Here's how the part is built. I have some questions about the finished solid (model axes, mm). A direction names the side the tool comes from. Round coordinates to 2 decimals unless told otherwise and drop trailing zeros. Loops run counter-clockwise (first coordinate to the right, second up) from the corner with the lowest first, then second, coordinate; pieces in that order, holes last. Notation, with made-up numbers: M -16,1 L 40,1 A16 ccw 40,17 Z; hole C 34.5,1 d9. An arc over 180 degrees is marked long. Answer as a JSON object with one key per item and string values.
from build123d import *

# Parameters (mm, degrees)
SKETCH1_R           = 2.1
SKETCH1_R_2         = 10
BOSS_EXTRUDE1_DEPTH = 6.35


with BuildPart() as part:
    # Sketch1 → Boss-Extrude1 (new body)
    with BuildSketch(Plane(origin=(0, 0, 0), x_dir=(1, 0, 0), z_dir=(0, 1, 0))):
        with BuildLine():
            ThreePointArc((-138, 42.5), (-180.5, 0), (-138, -42.5))
            Line((-138, -42.5), (0, -42.5))
            ThreePointArc((0, -42.5), (42.5, 0), (0, 42.5))
            Line((0, 42.5), (-138, 42.5))
        make_face()
        with BuildLine():
            Line((-103, 2.5), (-93, 2.5))
            ThreePointArc((-93, 2.5), (-90.5, 0), (-93, -2.5))
            Line((-93, -2.5), (-103, -2.5))
            ThreePointArc((-103, -2.5), (-105.5, 0), (-103, 2.5))
        make_face(mode=Mode.SUBTRACT)
        with BuildLine():
            ThreePointArc((-138, -37.5), (-140.5, -35), (-138, -32.5))
            Line((-138, -32.5), (-128, -32.5))
            ThreePointArc((-128, -32.5), (-125.5, -35), (-128, -37.5))
            Line((-128, -37.5), (-138, -37.5))
        make_face(mode=Mode.SUBTRACT)
        with BuildLine():
            ThreePointArc((-173, -2.5), (-175.5, 0), (-173, 2.5))
            Line((-173, 2.5), (-163, 2.5))
            ThreePointArc((-163, 2.5), (-160.5, 0), (-163, -2.5))
            Line((-163, -2.5), (-173, -2.5))
        make_face(mode=Mode.SUBTRACT)
        with BuildLine():
            ThreePointArc((-138, -10), (-148, 0), (-138, 10))
            Line((-138, 10), (-128, 10))
            ThreePointArc((-128, 10), (-118, 0), (-128, -10))
            Line((-128, -10), (-138, -10))
        make_face(mode=Mode.SUBTRACT)
        with BuildLine():
            ThreePointArc((-138, 32.5), (-140.5, 35), (-138, 37.5))
            Line((-138, 37.5), (-128, 37.5))
            ThreePointArc((-128, 37.5), (-125.5, 35), (-128, 32.5))
            Line((-128, 32.5), (-138, 32.5))
        make_face(mode=Mode.SUBTRACT)
        with Locations(Location((0, 35, 0), (0, 0, 270))):
            Circle(SKETCH1_R, mode=Mode.SUBTRACT)
        with Locations(Location((0, -35, 0), (0, 0, 270))):
            Circle(SKETCH1_R, mode=Mode.SUBTRACT)
        with Locations(Location((-17.67766953, -17.67766953, 0), (0, 0, 270))):
            Circle(SKETCH1_R, mode=Mode.SUBTRACT)
        with Locations(Location((17.67766953, -17.67766953, 0), (0, 0, 270))):
            Circle(SKETCH1_R, mode=Mode.SUBTRACT)
        with Locations(Location((-35, 0, 0), (0, 0, 270))):
            Circle(SKETCH1_R, mode=Mode.SUBTRACT)
        with Locations(Location((-17.67766953, 17.67766953, 0), (0, 0, 270))):
            Circle(SKETCH1_R, mode=Mode.SUBTRACT)
        with Locations(Location((0, 0, 0), (0, 0, 270))):
            Circle(SKETCH1_R_2, mode=Mode.SUBTRACT)
        with Locations(Location((35, 0, 0), (0, 0, 270))):
            Circle(SKETCH1_R, mode=Mode.SUBTRACT)
        with Locations(Location((17.67766953, 17.67766953, 0), (0, 0, 270))):
            Circle(SKETCH1_R, mode=Mode.SUBTRACT)
    extrude(amount=-BOSS_EXTRUDE1_DEPTH)


solid = part.part
Item 1: For faces 4 (the face through (-140.5, -3.1, 35.1)), 5 (the face through (-71, -6.35, -1)), which set-ups out of +Z, -Z, +X, -X, +Y, -Y let a thin tool reach every point of the face, with its end or its side?
Solution:
{"face 4": "+Y, -Y", "face 5": "+Z, -Z, +X, -X, -Y"}
Item 2: I want a section at A-A on z = 0. List the corners of the cut face in (x, y) for me, plus the area to 3 significant figures.
Solution:
{"outline": "M -180.5,-6.35 L -175.5,-6.35 L -175.5,0 L -180.5,0 Z; M -160.5,-6.35 L -148,-6.35 L -148,0 L -160.5,0 Z; M -118,-6.35 L -105.5,-6.35 L -105.5,0 L -118,0 Z; M -90.5,-6.35 L -37.1,-6.35 L -37.1,0 L -90.5,0 Z; M -32.9,-6.35 L -10,-6.35 L -10,0 L -32.9,0 Z; M 10,-6.35 L 32.9,-6.35 L 32.9,0 L 10,0 Z; M 37.1,-6.35 L 42.5,-6.35 L 42.5,0 L 37.1,0 Z", "area": "855 mm2"}
Item 3: If I drill on L1, parallel to X at y = -3.5, z = 7.5; L2, parallel to X at y = -1.5, z = 3; L3, parallel to Z at x = -147, y = -2.25, over which ranges is the centre line in solid material (lowest first)? Write a range as from..to.
Solution:
{"L1": "x = -179.83..-144.61, -121.39..-6.61, 6.61..41.83", "L2": "x = -180.39..-147.54, -118.46..-9.54, 9.54..42.39", "L3": "z = -41.54..-4.36, 4.36..41.54"}
Item 4: We'd pull the mould along Z, two halves only. Please class faces 1 (the face through (-71, 0, -1)), 2 (the face through (0.09, -3.13, 32.9)), 3 (the face through (-180.49, -3.13, -0.93)): +Z half, -Z half, draft (parallel to the pull), parting line (faces both ways), or undercut.
Solution:
{"face 1": "draft", "face 2": "undercut", "face 3": "parting line"}
Item 5: For P1, Ø1, axis at y = -4, z = -16.5, coming from the +X side; P2, Ø1.9, axis at x = -167.5, y = -3.5, coming from the -Z side, each with a flat end and sliding along its axis, tell me the tip position at first contact or that it passes through.
Solution:
{"P1": "stops at x = 39.37", "P2": "stops at z = -31.48"}
Item 6: I want a section at D-D on z = 35. List the corners of the cut face in (x, y) for me.
Solution:
{"outline": "M -162.11,-6.35 L -140.5,-6.35 L -140.5,0 L -162.11,0 Z; M -125.5,-6.35 L -2.1,-6.35 L -2.1,0 L -125.5,0 Z; M 2.1,-6.35 L 24.11,-6.35 L 24.11,0 L 2.1,0 Z"}
Item 7: I want a section at B-B on x = -97.5. List the corners of the cut face in (y, z) for me, plus the area to 3 significant figures.
Solution:
{"outline": "M -6.35,-42.5 L 0,-42.5 L 0,-2.5 L -6.35,-2.5 Z; M -6.35,2.5 L 0,2.5 L 0,42.5 L -6.35,42.5 Z", "area": "508 mm2"}
Item 8: I want a section at C-C on x = -136. List the corners of the cut face in (y, z) for me.
Solution:
{"outline": "M -6.35,-42.5 L 0,-42.5 L 0,-37.5 L -6.35,-37.5 Z; M -6.35,-32.5 L 0,-32.5 L 0,-10 L -6.35,-10 Z; M -6.35,10 L 0,10 L 0,32.5 L -6.35,32.5 Z; M -6.35,37.5 L 0,37.5 L 0,42.5 L -6.35,42.5 Z"}
